Source: three-view drawing plus pictorial views. Frame: mm from the lowest corner of the part. A direction names the side the tool comes from. Give positions to 0.01 mm unless a question says otherwise; leave off trailing zeros. Loops run counter-clockwise (first coordinate to the right, second up) from the corner with the lowest first, then second, coordinate; pieces in that order, holes last.
1. Material intervals for line 1 along Y through (x, z) = (5.5, 5.5); line 2 along Z through (x, y) = (9, 18.75); line 3 along Y through (x, z) = (6, 1), sorted ascending.
2. Section A-A, the plane y = 9. Output: boundary loops of the cut face in (x, z).
3. First-contact query: P1, Ø8, axis at y = 11, z = 7, coming from the +X side (1 decimal); P2, Ø2, axis at x = 11.5, y = 16, coming from the -Z side; P3, Ø8, axis at x = 1.5, y = 10, coming from the -Z side; P4, Ø5, axis at x = 8.5, y = 17, coming from the -Z side. Flat tips, straight axial feed; report the tip coordinate or a pass-through.
4. Access query for the marked faces 1, 2 and 3. Directions: +Z, -Z, +X, -X, +Y, -Y. A direction counts if a zero-diameter tool reaches every point of the face in a straight line with its end or side. Return the directions, or none.
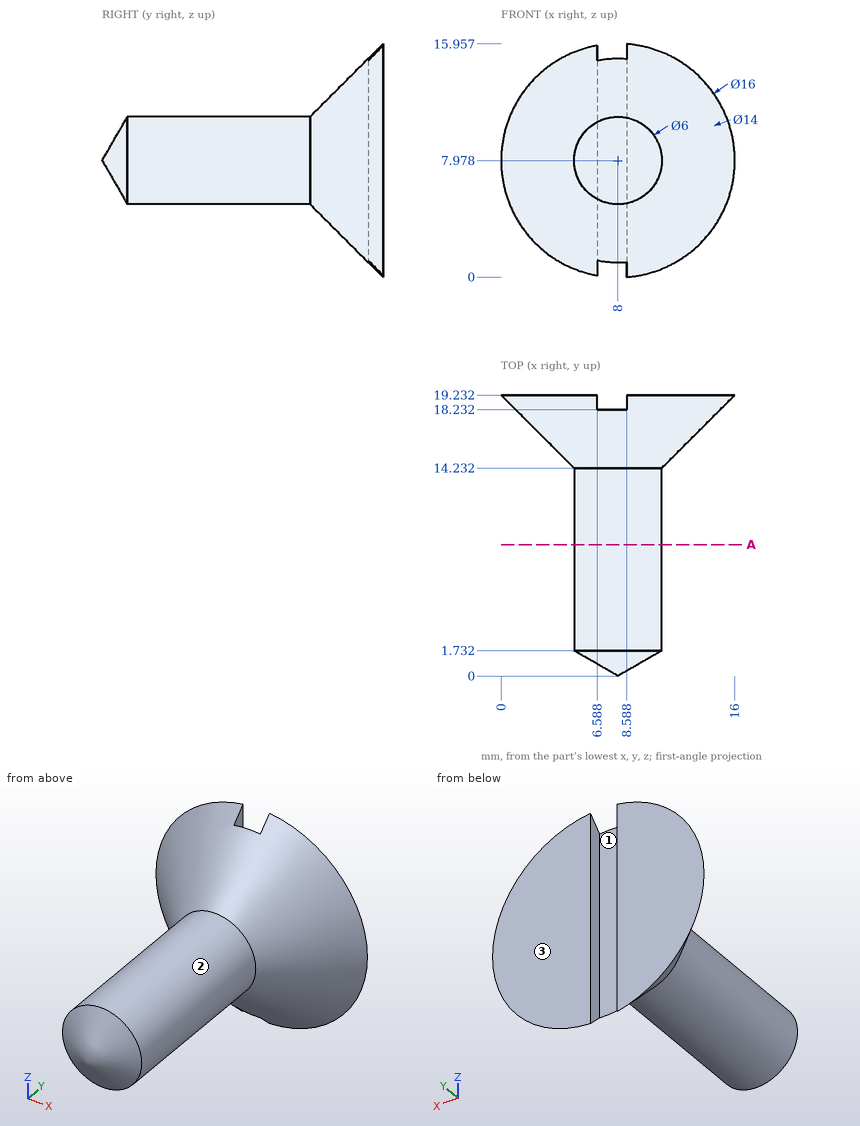
Answers below:
1. line 1: y = 14.75 to 19.23
1. line 2: z = 0.53 to 15.43
1. line 3: y = 18.49 to 19.23
2. outline: circle Ø6 at (8, 7.98)
3. P1: stops at x = 11.7
3. P2: stops at z = 3.21
3. P3: stops at z = 6.32
3. P4: stops at z = 0
4. face 1: +Z, -Z, +Y
4. face 2: -Y
4. face 3: +Z, -Z, +X, -X, +Y
